```python
from build123d import *

# Parameters (mm, degrees)
ESBO_O1_W                = 7
ESBO_O1_H                = 33
ESBO_O1_R                = 1.65
RESSALTO_EXTRUS_O1_DEPTH = 4
ESBO_O2_W                = 0.6
ESBO_O2_H                = 6.5
CORTE_EXTRUS_O1_DEPTH    = 8


with BuildPart() as part:
    # Esboço1 → Ressalto-extrusão1 (new body)
    with BuildSketch(Plane.XY):
        Rectangle(ESBO_O1_W, ESBO_O1_H)
        Circle(ESBO_O1_R, mode=Mode.SUBTRACT)
        with Locations((0, 12.5)):
            Circle(ESBO_O1_R, mode=Mode.SUBTRACT)
        with Locations((0, -12.5)):
            Circle(ESBO_O1_R, mode=Mode.SUBTRACT)
    extrude(amount=RESSALTO_EXTRUS_O1_DEPTH)

    # Esboço2 → Corte-extrusão1 (cut, through all)
    with BuildSketch(Plane.ZY.offset(3.5)):
        with Locations((0.3, 6.75)):
            Rectangle(ESBO_O2_W, ESBO_O2_H)
        with Locations((0.3, -6.75)):
            Rectangle(ESBO_O2_W, ESBO_O2_H)
    extrude(amount=-CORTE_EXTRUS_O1_DEPTH, mode=Mode.SUBTRACT)


solid = part.part
```
Geometry check sheet. Reference: the model listing, model coordinates, mm. A direction names the side the tool comes from. Give positions to 0.01 mm unless a question says otherwise; leave off trailing zeros. Write each loop counter-clockwise with the first axis right and the second up, starting at its lowest first coordinate (ties: lowest second). Pieces come first, ordered by that corner, then holes.
1) Gauge pin test, flat end, axial feed: pin 1 (2 mm diameter, centred on x = 1.5, y = 6, fed in from -Z). Record the tip position at first contact, or that the pin passes through.
2) Release check for a two-part mould opening along Y. For faces 3 (the flat face through (-2, 1, 0)), 4 (the cylindrical face through (-0.4, -14.1, 2)), 5 (the flat face through (0, 16.5, 2)) record: pulls with the +Y half, pulls with the -Y half, needs draft (parallel to the pull), parting line crosses it, or undercut.
3) Section check D-D, the plane x = -2.75. Record the boundary of the cut face in (y, z), and give its area (3 significant figures).
4) Access from +Z, -Z, +X, -X, +Y, -Y to the whole of each face (thin tool, end or side, straight path). Record for faces 1 (the flat face through (0, -15, 0)), 2 (the flat face through (0, -7, 0.6)).
5) Section check A-A, the plane x = 0. Record the boundary of the cut face in (y, z), and give its area (3 significant figures).
6) Section check B-B, the plane y = -12.5. Record the boundary of the cut face in (x, z), and give its area (3 significant figures).
7) Section check C-C, the plane z = 1.8. Record the boundary of the cut face in (x, y).
8) Material ranges on L1, parallel to Y at x = 0, z = 1.85; L2, parallel to Y at x = 3, z = 0.4; L3, parallel to Y at x = -1.25, z = 2, recorded low to high.
Computed:
1. pin 1: stops at z = 0.6
2. face 3: needs draft
2. face 4: undercut
2. face 5: pulls with the +Y half
3. outline: (-16.5, 0) - (-10, 0) - (-10, 0.6) - (-3.5, 0.6) - (-3.5, 0) - (3.5, 0) - (3.5, 0.6) - (10, 0.6) - (10, 0) - (16.5, 0) - (16.5, 4) - (-16.5, 4) - close
3. area: 124 mm2
4. face 1: -Z, +X, -X, +Y, -Y
4. face 2: -Z, +X, -X
5. outline: (-16.5, 0) - (-14.15, 0) - (-14.15, 4) - (-16.5, 4) - close; (-10.85, 0) - (-10, 0) - (-10, 0.6) - (-3.5, 0.6) - (-3.5, 0) - (-1.65, 0) - (-1.65, 4) - (-10.85, 4) - close; (1.65, 0) - (3.5, 0) - (3.5, 0.6) - (10, 0.6) - (10, 0) - (10.85, 0) - (10.85, 4) - (1.65, 4) - close; (14.15, 0) - (16.5, 0) - (16.5, 4) - (14.15, 4) - close
5. area: 84.6 mm2
6. outline: (-3.5, 0) - (-1.65, 0) - (-1.65, 4) - (-3.5, 4) - close; (1.65, 0) - (3.5, 0) - (3.5, 4) - (1.65, 4) - close
6. area: 14.8 mm2
7. outline: (-3.5, -16.5) - (3.5, -16.5) - (3.5, 16.5) - (-3.5, 16.5) - close; hole circle Ø3.3 at (0, -12.5); hole circle Ø3.3 at (0, 0); hole circle Ø3.3 at (0, 12.5)
8. L1: y = -16.5 to -14.15, -10.85 to -1.65, 1.65 to 10.85, 14.15 to 16.5
8. L2: y = -16.5 to -10, -3.5 to 3.5, 10 to 16.5
8. L3: y = -16.5 to -13.58, -11.42 to -1.08, 1.08 to 11.42, 13.58 to 16.5
